Geometry: final body of the model. Coordinates: model frame, mm. A direction names the side the tool comes from. Give positions to 0.01 mm unless a question says otherwise; leave off trailing zeros.
1. Material intervals for line 1 along X through (y, z) = (-0.25, 3.75); line 2 along Z through (x, y) = (184.15, 0); line 3 along Z through (x, y) = (204, 5.5), sorted ascending.
2. Access query for faces 1 (the face through (-378.46, 0, 6)), 2 (the face through (10, 0, -6.35)), 3 (the face through (-74, 4, -3.175)). Directions: +Z, -Z, +X, -X, +Y, -Y. A direction counts if a zero-diameter tool reaches every point of the face in a straight line with its end or side. Return the directions, or none.
3. First-contact query: P1, Ø0.9, axis at x = -184.5, z = 0.5, coming from the +Y side; P2, Ø1.1, axis at y = -0.5, z = 1, coming from the +X side; P3, Ø4, axis at x = -203.2, z = 0, coming from the -Y side. Flat tips, straight axial feed; report the tip coordinate or a pass-through.
4. Draft query along X for faces 4 (the face through (-74, 4, 3.175)), 5 (the face through (387.35, 0, -6)), 6 (the face through (10, 0, 6.35)). Return one class per face: +X half, -X half, draft (parallel to the pull), parting line (faces both ways), or undercut.
from build123d import *

# Parameters (mm, degrees)
SKETCH1_W                       = 12.7
SKETCH1_H                       = 12.82133758
LENGTH_DEPTH                    = 406.4
SKETCH2_W                       = 12.7
SKETCH2_H                       = 12.82133758
SKETCH2_R                       = 5.334
ROUND_CUT_1_DEPTH               = 19.05
SKETCH3_W                       = 12.7
SKETCH3_H                       = 12.82133758
SKETCH3_R                       = 5.334
ROUND_CUT_2_DEPTH               = 27.94
SKETCH14_R                      = 1.7526
CUT_EXTRUDE6_DEPTH              = 12.7
SKETCH15_R                      = 1.7526
CUT_EXTRUDE7_DEPTH              = 19.05
BOTTOM_WASHER_R                 = 1.4224
BOTTOM_WASHER_BOLTS_DEPTH       = 10.922
BOTTOM_WASHER_CENTER_BOLT_REACH = 14.821
SKETCH18_R                      = 3.175
TOP_WASHER_CENTER_BOLT_REACH    = 14.821
SKETCH17_R                      = 3.175
SKETCH16_R                      = 1.4224
TOP_WASHER_DEPTH                = 10.922
SKETCH19_W                      = 69.85
SKETCH19_H                      = 6.35
CUT_EXTRUDE8_DEPTH              = 13.82133758
SKETCH20_R                      = 1.397
SKETCH20_R_2                    = 3.175
CUT_EXTRUDE9_DEPTH              = 13.7


with BuildPart() as part:
    # Sketch1 → Length (new body, symmetric)
    with BuildSketch(Plane(origin=(0, 0, 0), x_dir=(0, 0, -1), z_dir=(1, 0, 0))):
        Rectangle(SKETCH1_W, SKETCH1_H)
    extrude(amount=LENGTH_DEPTH, both=True)

    # Sketch2 → Round Cut 1 (cut)
    with BuildSketch(Plane(origin=(406.4, 0, 0), x_dir=(0, 0, -1), z_dir=(1, 0, 0))):
        Rectangle(SKETCH2_W, SKETCH2_H)
        Circle(SKETCH2_R, mode=Mode.SUBTRACT)
    extrude(amount=-ROUND_CUT_1_DEPTH, mode=Mode.SUBTRACT)

    # Sketch3 → Round Cut 2 (cut)
    with BuildSketch(Plane.ZY.offset(406.4)):
        Rectangle(SKETCH3_W, SKETCH3_H)
        Circle(SKETCH3_R, mode=Mode.SUBTRACT)
    extrude(amount=-ROUND_CUT_2_DEPTH, mode=Mode.SUBTRACT)

    # Sketch14 → Cut-Extrude6 (cut)
    with BuildSketch(Plane(origin=(406.4, 0, 0), x_dir=(0, 0, -1), z_dir=(1, 0, 0))):
        Circle(SKETCH14_R)
    extrude(amount=-CUT_EXTRUDE6_DEPTH, mode=Mode.SUBTRACT)

    # Sketch15 → Cut-Extrude7 (cut)
    with BuildSketch(Plane.ZY.offset(406.4)):
        Circle(SKETCH15_R)
    extrude(amount=-CUT_EXTRUDE7_DEPTH, mode=Mode.SUBTRACT)

    # Bottom Washer → Bottom washer bolts (cut)
    with BuildSketch(Plane(origin=(0, 6.41066879, 0), x_dir=(1, 0, 0), z_dir=(0, 1, 0))):
        with Locations((-222.25, 0)):
            Circle(BOTTOM_WASHER_R)
        with Locations((-184.15, 0)):
            Circle(BOTTOM_WASHER_R)
    extrude(amount=-BOTTOM_WASHER_BOLTS_DEPTH, mode=Mode.SUBTRACT)

    # Sketch18 → Bottom Washer Center Bolt (cut, up to next)
    with BuildSketch(Plane(origin=(0, 6.41066879, 0), x_dir=(1, 0, 0), z_dir=(0, 1, 0)), mode=Mode.PRIVATE) as bottom_washer_center_bolt_sk1:
        with Locations((-203.2, 0)):
            Circle(SKETCH18_R)
    bottom_washer_center_bolt_tool1 = extrude(bottom_washer_center_bolt_sk1.sketch, amount=-BOTTOM_WASHER_CENTER_BOLT_REACH, mode=Mode.PRIVATE) & part.part
    add(bottom_washer_center_bolt_tool1.solids().sort_by_distance((-203.2, 6.410669, 0))[0], mode=Mode.SUBTRACT)

    # Sketch17 → Top Washer Center Bolt (cut, up to next)
    with BuildSketch(Plane(origin=(0, 6.41066879, 0), x_dir=(1, 0, 0), z_dir=(0, 1, 0)), mode=Mode.PRIVATE) as top_washer_center_bolt_sk1:
        with Locations((203.2, 0)):
            Circle(SKETCH17_R)
    top_washer_center_bolt_tool1 = extrude(top_washer_center_bolt_sk1.sketch, amount=-TOP_WASHER_CENTER_BOLT_REACH, mode=Mode.PRIVATE) & part.part
    add(top_washer_center_bolt_tool1.solids().sort_by_distance((203.2, 6.410669, 0))[0], mode=Mode.SUBTRACT)

    # Sketch16 → Top Washer (cut)
    with BuildSketch(Plane(origin=(0, 6.41066879, 0), x_dir=(1, 0, 0), z_dir=(0, 1, 0))):
        with Locations((222.25, 0)):
            Circle(SKETCH16_R)
        with Locations((184.15, 0)):
            Circle(SKETCH16_R)
    extrude(amount=-TOP_WASHER_DEPTH, mode=Mode.SUBTRACT)

    # Sketch19 → Cut-Extrude8 (cut, through all)
    with BuildSketch(Plane(origin=(0, -6.41066879, 0), x_dir=(-1, 0, 0), z_dir=(0, -1, 0))):
        with Locations((74.285606639, 0)):
            Rectangle(SKETCH19_W, SKETCH19_H)
    extrude(amount=-CUT_EXTRUDE8_DEPTH, mode=Mode.SUBTRACT)

    # Sketch20 → Cut-Extrude9 (cut, through all)
    with BuildSketch(Plane.XY.offset(6.35)):
        with Locations((-93.335606639, 0)):
            Circle(SKETCH20_R)
        with Locations((-74.285606639, 0)):
            Circle(SKETCH20_R_2)
        with Locations((-55.235606639, 0)):
            Circle(SKETCH20_R)
    extrude(amount=-CUT_EXTRUDE9_DEPTH, mode=Mode.SUBTRACT)


solid = part.part
Answers below:
1. line 1: x = -406.4 to -94.71, -91.96 to -77.45, -71.12 to -56.61, -53.86 to 406.4
1. line 2: z = -6.35 to -1.42, 1.42 to 6.35
1. line 3: z = -6.35 to -3.07, 3.07 to 6.35
2. face 1: -X
2. face 2: -Z, +X, -X, +Y, -Y
2. face 3: +Y, -Y
3. P1: stops at y = -4.51
3. P2: stops at x = 393.7
3. P3: passes through
4. face 4: undercut
4. face 5: +X half
4. face 6: draft
